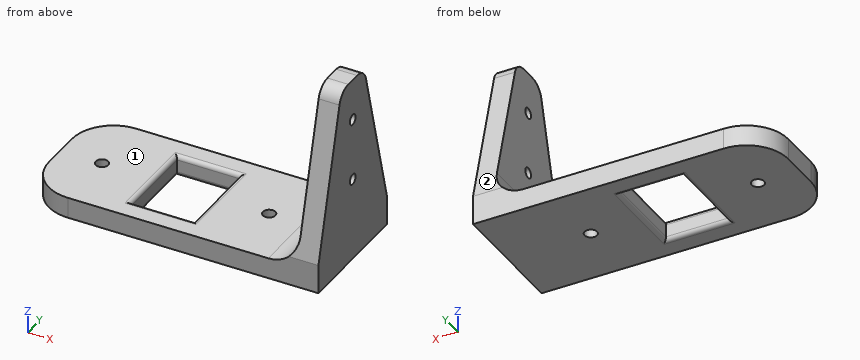
from build123d import *

# Parameters (mm, degrees)
SKETCH_W      = 70
SKETCH_H      = 30
SKETCH_R      = 1.5
SKETCH_W_2    = 15
SKETCH_H_2    = 20
PAD_DEPTH     = 5
FILLET_R      = 10
FILLET001_R   = 1
SKETCH001_W   = 5
SKETCH001_H   = 30
PAD001_DEPTH  = 40
CHAMFER_SIZE2 = 38
CHAMFER_SIZE  = 10
FILLET002_R   = 7
SKETCH002_R   = 1.25
POCKET_DEPTH  = 70.001
FILLET003_R   = 4


with BuildPart() as part:
    # Sketch → Pad (new body)
    with BuildSketch(Plane.XY):
        with Locations((25, 0)):
            Rectangle(SKETCH_W, SKETCH_H)
        Circle(SKETCH_R, mode=Mode.SUBTRACT)
        with Locations((40, 0)):
            Circle(SKETCH_R, mode=Mode.SUBTRACT)
        with Locations((20, 0)):
            Rectangle(SKETCH_W_2, SKETCH_H_2, mode=Mode.SUBTRACT)
    extrude(amount=PAD_DEPTH)

    # Fillet
    fillet_edges = [part.edges().sort_by_distance(p)[0] for p in [
        (-10, 15, 2.5),
        (-10, -15, 2.5),
    ]]
    fillet(fillet_edges, radius=FILLET_R)

    # Fillet001
    fillet001_edges = [part.edges().sort_by_distance(p)[0] for p in [
        (12.5, 0, 5),
        (12.5, 0, 0),
        (20, 10, 0),
        (20, 10, 5),
        (27.5, 0, 5),
        (20, -10, 5),
        (27.5, 0, 0),
        (20, -10, 0),
    ]]
    fillet(fillet001_edges, radius=FILLET001_R)

    # Sketch001 (on Face18 of Fillet001) → Pad001 (join)
    with BuildSketch(Plane.XY.offset(5)):
        with Locations((57.5, 0)):
            Rectangle(SKETCH001_W, SKETCH001_H)
    extrude(amount=PAD001_DEPTH)

    # Chamfer
    chamfer_edges = [part.edges().sort_by_distance(p)[0] for p in [
        (57.5, -15, 45),
        (57.5, 15, 45),
    ]]
    chamfer_side = part.faces().sort_by_distance((57.5, 0, 45))[0]
    chamfer(chamfer_edges, length=CHAMFER_SIZE, length2=CHAMFER_SIZE2, reference=chamfer_side)

    # Fillet002
    fillet002_edges = [part.edges().sort_by_distance(p)[0] for p in [
        (55, 0, 5),
    ]]
    fillet(fillet002_edges, radius=FILLET002_R)

    # Sketch002 (on Face7 of Fillet002) → Pocket (cut, through all)
    with BuildSketch(Plane.YZ.offset(60)):
        with Locations((0, 35)):
            Circle(SKETCH002_R)
        with Locations((0, 20)):
            Circle(SKETCH002_R)
    extrude(amount=-POCKET_DEPTH, mode=Mode.SUBTRACT)

    # Fillet003
    fillet003_edges = [part.edges().sort_by_distance(p)[0] for p in [
        (57.5, 5, 45),
        (57.5, -5, 45),
    ]]
    fillet(fillet003_edges, radius=FILLET003_R)


solid = part.part
Build history of the part. All positions in model axes, mm. Face numbers are marked on the shaded views. A direction names the side the tool comes from. Coordinates: 2 decimals unless noted, no trailing zeros. Write each loop counter-clockwise with the first axis right and the second up, starting at its lowest first coordinate (ties: lowest second). Pieces come first, ordered by that corner, then holes.
(1) Drill centre lines: line 1 (Z direction, x = 57, y = 0); line 2 (Z direction, x = 6.5, y = 10); line 3 (Y direction, x = 40, z = 1). Where is each one in solid material? Low to high.
(2) Pin check, flat tips, straight feed: pin 1 Ø5 at (x, y) = (40, 0) entering from +Z; pin 2 Ø6 at (y, z) = (10.5, 7.5) entering from -X. Stop position of each tip, or through.
(3) Cut at C-C on z = 20. List the corners of the cut face in (x, y), and give its area (3 significant figures).
(4) Cut at A-A on x = 40. List the corners of the cut face in (y, z).
(5) Cut at B-B on y = 0. State how many separate pieces and enclosed holes the cut face has, and give its area (3 significant figures).
(6) 3-axis set-ups, long thin cutter, end or side, ignore diameter. For the marked faces 1 and 2: which of +Z, -Z, +X, -X, +Y, -Y reach the whole face in a straight line?
(7) Cut at D-D on y = 12. List the corners of the cut face in (x, z), and give its area (3 significant figures).
Working result:
1. line 1: z = 0 to 18.75, 21.25 to 33.75, 36.25 to 45
1. line 2: z = 0 to 5
1. line 3: y = -15 to -1.5, 1.5 to 15
2. pin 1: stops at z = 5
2. pin 2: stops at x = -9.23
3. outline: (55, -11.58) - (60, -11.58) - (60, -1.25) - (55, -1.25) - close; (55, 1.25) - (60, 1.25) - (60, 11.58) - (55, 11.58) - close
3. area: 103 mm2
4. outline: (-15, 0) - (-1.5, 0) - (-1.5, 5) - (-15, 5) - close; (1.5, 0) - (15, 0) - (15, 5) - (1.5, 5) - close
5. separate pieces: 6
5. enclosed holes: 0
5. area: 430 mm2
6. face 1: +Z, -X, +Y, -Y
6. face 2: +Z, +X, -X, +Y
7. outline: (-7.14, 0) - (60, 0) - (60, 18.4) - (55, 18.4) - (55, 12) arc R7 cw to (48, 5) - (-7.14, 5) - close
7. area: 413 mm2
